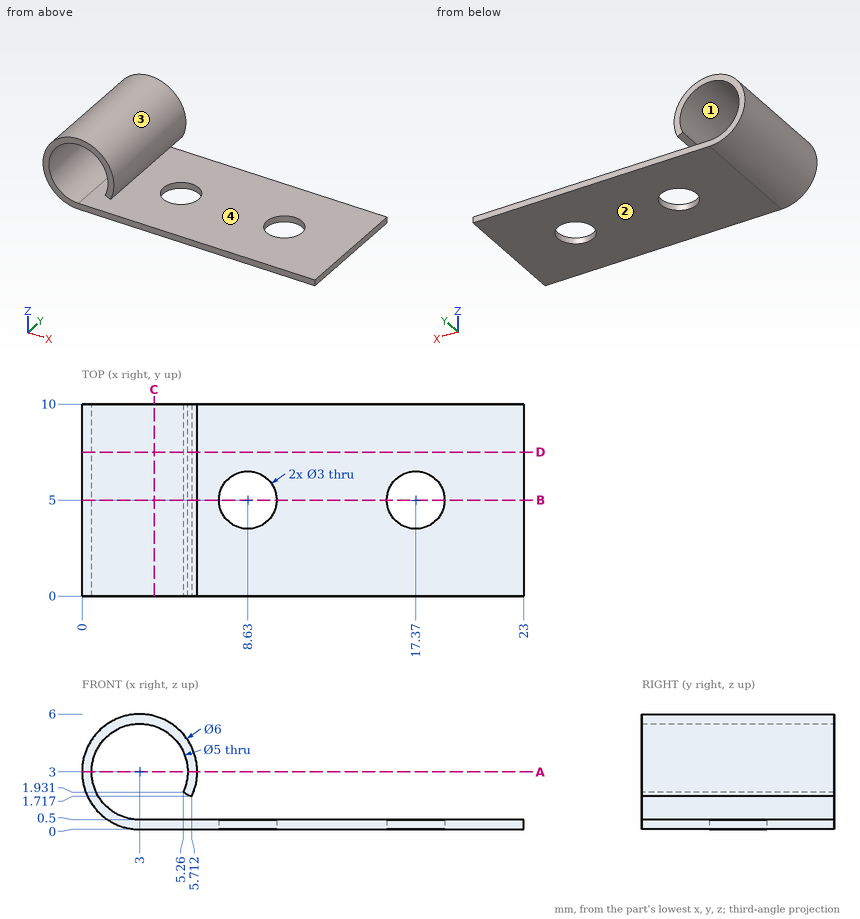
Part print with two shaded views. Sizes in mm from the minimum x, y, z corner. A direction names the side the tool comes from. Coordinates: 2 decimals unless noted, no trailing zeros. Write each loop counter-clockwise with the first axis right and the second up, starting at its lowest first coordinate (ties: lowest second). Pieces come first, ordered by that corner, then holes. Notation, with made-up numbers: (51.25, 6.25) - (60.25, 6.25) arc R25 ccw to (60.25, 41.25) - close; hole circle Ø5 at (74, 27). An arc over 180 degrees is marked (long way). Put each result on its own line as item: value.
1. Band-saw the part on A-A (z = 3). Write the cut outline in (x, y), then the cut area to 3 significant figures.
Final values:
outline: (0, 0) - (0.5, 0) - (0.5, 10) - (0, 10) - close; (5.5, 0) - (6, 0) - (6, 10) - (5.5, 10) - close
area: 10.0 mm²
2. Two-plate mould, pull along Z, no slides. Class the marked faces 1 and 2: +Z half, -Z half, draft (parallel to the pull), parting line (faces both ways), or undercut.
Final values:
face 1: undercut
face 2: -Z half
3. Band-saw the part on D-D (y = 7.5). Write the cut outline in (x, z).
Final values:
outline: (3, 0) - (23, 0) - (23, 0.5) - (3, 0.5) arc R2.5 cw (long way) to (5.26, 1.93) - (5.71, 1.72) arc R3 ccw (long way) to start
4. Band-saw the part on B-B (y = 5). Write the cut outline in (x, z).
Final values:
outline: (3, 0) - (7.13, 0) - (7.13, 0.5) - (3, 0.5) arc R2.5 cw (long way) to (5.26, 1.93) - (5.71, 1.72) arc R3 ccw (long way) to start; (10.13, 0) - (15.87, 0) - (15.87, 0.5) - (10.13, 0.5) - close; (18.87, 0) - (23, 0) - (23, 0.5) - (18.87, 0.5) - close
5. 3-axis set-ups, long thin cutter, end or side, ignore diameter. For the marked faces 3 and 4: which of +Z, -Z, +X, -X, +Y, -Y reach the whole face in a straight line?
Final values:
face 3: +Y, -Y
face 4: +X, +Y, -Y
6. Flat gauge pin, fed straight in: pin 1 Ø5 at (x, y) = (14.5, 5) entering from +Z. Where does the tip first touch, or does it go through?
Final values:
pin 1: stops at z = 0.5
7. Probe line 1 along X through (y, z) = (4.75, 3); line 2 along Z through (x, y) = (21, 3.25); line 3 along X through (y, z) = (2.5, 5.25) (1 decimal). List the from-to ranges inside material, lowest first. Write a range as [from, to].
Final values:
line 1: x = [0, 0.5], [5.5, 6]
line 2: z = [0, 0.5]
line 3: x = [1, 1.9], [4.1, 5]
8. Band-saw the part on C-C (x = 3.75). Write the cut outline in (y, z) (1 decimal).
Final values:
outline: (0, 0) - (10, 0) - (10, 0.5) - (0, 0.5) - close; (0, 5.4) - (10, 5.4) - (10, 5.9) - (0, 5.9) - close
